```python
from build123d import *

# Parameters (mm, degrees)
BASPROSKE_W      = 5
BASPROSKE_H      = 5.5
TOOTHCUT_DEPTH   = 10.246621004
TEETHCUTS_COUNT  = 20
TEETHCUTS_ANGLE  = 342
HUBNEAONESKE_R   = 4
HUBNEARONE_DEPTH = 5.0000508
BORSKE_R         = 0.4
BORE_DEPTH       = 10.0000508


with BuildPart() as part:
    # BasProSke → Base-Revolve (revolve)
    with BuildSketch(Plane(origin=(0, 0, 0), x_dir=(1, 0, 0), z_dir=(0, 1, 0)), mode=Mode.PRIVATE) as base_revolve_sk:
        with Locations((2.5, 2.75)):
            Rectangle(BASPROSKE_W, BASPROSKE_H)
    revolve(base_revolve_sk.sketch.rotate(Axis((-10, 0, 0), (1, 0, 0)), 180), axis=Axis((-10, 0, 0), (1, 0, 0)))

    # TooCutSke → ToothCut (cut, through all)
    with BuildSketch(Plane(origin=(0, 0, 0), x_dir=(0, 0, -1), z_dir=(1, 0, 0))):
        with BuildLine():
            ThreePointArc((0.249903181, 4.366855207), (0, 4.374), (-0.249903181, 4.366855207))
            ThreePointArc((-0.249903181, 4.366855207), (-0.415207844, 4.95951031), (-0.752843848, 5.473871692))
            ThreePointArc((-0.752843848, 5.473871692), (0, 5.5254), (0.752843848, 5.473871692))
            ThreePointArc((0.752843848, 5.473871692), (0.415207844, 4.95951031), (0.249903181, 4.366855207))
        make_face()
    toothcut = extrude(amount=TOOTHCUT_DEPTH, mode=Mode.SUBTRACT)

    # TeethCuts: ToothCut ×20 about axis
    teethcuts_axis = Axis((-10, 0, 0), (1, 0, 0))
    for i in range(1, TEETHCUTS_COUNT):
        add(toothcut.rotate(teethcuts_axis, i * TEETHCUTS_ANGLE / (TEETHCUTS_COUNT - 1)), mode=Mode.SUBTRACT)

    # HubNeaOneSke → HubNearOne (add)
    with BuildSketch(Plane.ZY):
        with Locations(Location((0, 0, 0), (0, 0, 180))):
            Circle(HUBNEAONESKE_R)
    extrude(amount=HUBNEARONE_DEPTH)

    # BorSke → Bore (cut, symmetric)
    with BuildSketch(Plane(origin=(0, 0, 0), x_dir=(0, 0, -1), z_dir=(1, 0, 0))):
        with Locations(Location((0, 0, 0), (0, 0, 180))):
            Circle(BORSKE_R)
    extrude(amount=BORE_DEPTH, both=True, mode=Mode.SUBTRACT)


solid = part.part
```
Geometry: final body of the model. Coordinates: model frame, mm. A direction names the side the tool comes from. Round coordinates to 2 decimals unless told otherwise and drop trailing zeros. Order: outer loops, then holes, each group sorted by start corner. A loop starts at its lowest first (then second) coordinate and runs counter-clockwise, first axis right, second up. Notation, with made-up numbers: M -7,-36 L 41,-36 A20 ccw 41,-16 Z; hole C -14.5,13 d6. An arc over 180 degrees is marked long. Use one line per item in the form item = value. Start each with the question number.
Q1. Cut plane D-D (y = 1.75). Return loops of the section in (x, z), and give its area (3 significant figures).
Q2. Pin query (flat end, axial travel): pin 1 Ø2 at (x, y) = (1.5, 3) entering from -Z. Return the tip coordinate at first contact, or that it passes through.
Q3. Access query for faces 4 (the face through (2.46, 1.14, -4.84)), 5 (the face through (2.465, 0.406, -4.938)), 6 (the face through (2.46, 4.57, 1.91)). Directions: +Z, -Z, +X, -X, +Y, -Y. A direction counts if a zero-diameter tool reaches every point of the face in a straight line with its end or side. Return the directions, or none.
Q4. Material intervals for line 1 (Y direction, x = 1.75, z = 3.5); line 2 (Y direction, x = -0.5, z = 0), sorted ascending. Write a range as [from, to].
Q5. Cut plane A-A (y = 0). Return loops of the section in (x, z).
Q6. Mould query, pull axis Y, two halves, no side actions, for faces 1 (the face through (2.465, 3.245, 3.765)), 2 (the face through (-2.465, 3.905, 0.867)), 3 (the face through (2.465, 3.765, -3.245)). Classes: +Y half, -Y half, draft (parallel to the pull), parting line (faces both ways), or undercut.
Q7. Cut plane C-C (x = -3). Return loops of the section in (y, z), and give its area (3 significant figures).
Geometry results:
q1.outline = M -5,-3.6 L 0,-3.6 L 0,-4.36 L 5,-4.36 L 5,4.36 L 0,4.36 L 0,3.6 L -5,3.6 Z
q1.area = 79.6 mm^2
q2.pin_1 = -4.96
q3.face_4 = +X, -X
q3.face_5 = -Z, +X, -X
q3.face_6 = +X, -X, +Y
q4.line_1 = [-3.89, -2.88], [-2.62, 2.62], [2.88, 3.89]
q4.line_2 = [-4, -0.4], [0.4, 4]
q5.outline = M -5,-4 L 0,-4 L 0,-4.37 L 5,-4.37 L 5,-0.4 L -5,-0.4 Z; M -5,0.4 L 5,0.4 L 5,4.37 L 0,4.37 L 0,4 L -5,4 Z
q6.face_1 = undercut
q6.face_2 = parting line
q6.face_3 = +Y half
q7.outline = C 0,0 d8; hole C 0,0 d0.8
q7.area = 49.8 mm^2
